Check sheet for the modelled part. Datum: model origin and axes. Units: mm. A direction names the side the tool comes from. Give positions to 0.01 mm unless a question says otherwise; leave off trailing zeros. Write each loop counter-clockwise with the first axis right and the second up, starting at its lowest first coordinate (ties: lowest second). Pieces come first, ordered by that corner, then holes. Notation, with made-up numbers: M 67.25,-3.75 L 81.25,-3.75 A20 ccw 81.25,25.25 Z; hole C 24,-20 d1. An arc over 180 degrees is marked long. Use CSV: the item, a comma, the result in double quotes. Start each with the question number.
1. Scan lines: line 1 (Z direction, x = -15, y = -0.05); line 2 (X direction, y = -0.25, z = -29); line 3 (X direction, y = -0.3, z = -2). Record each from-to range of solid material in increasing order.
2. Cross-section at C-C, the plane y = 0.45. Enter the section's corners in (x, z).
3. Cross-section at B-B, the plane z = -35. Enter the section's corners in (x, y), and give its area (3 significant figures).
4. Cross-section at D-D, the plane z = 21. Enter the section's corners in (x, y).
5. Access from +Z, -Z, +X, -X, +Y, -Y to the whole of each face (thin tool, end or side, straight path). Record for faces 1 (the face through (-0.476, 0.493, 49.697)), 2 (the face through (27.75, -0.25, 34.94)), 3 (the face through (-5.43, -0.25, 46.97)).
6. Mould release check, pull along Z, two halves, no side actions. Record for faces 4 (the face through (-2, -0.5, 1)), 5 (the face through (23.274, -0.092, -0.447)), 6 (the face through (0.5, 0.5, -49.8)): +Z half, -Z half, draft (parallel to the pull), parting line (faces both ways), or undercut.
7. Cross-section at A-A, the plane x = -23. Enter the section's corners in (y, z).
8. Depth check by flat-ended pin: P1, Ø5, axis at x = 30.5, z = -35, coming from the -Y side; P2, Ø0.6, axis at y = -0.5, z = 31.5, coming from the +X side; P3, Ø8, axis at x = 26.5, z = -6, coming from the -Y side. Enter the tip coordinate at first touch or a pass-through.
from build123d import *

# Parameters (mm, degrees)
EXTRUDE_1_DEPTH     = 1
CUT_EXTRUDE_1_REACH = 65.213
SKETCH_3_R          = 1.5
EXTRUDE_2_DEPTH     = 0.5
FILLET_1_R          = 2


with BuildPart() as part:
    # 스케치2 → 보스-돌출1 (new body)
    with BuildSketch(Plane(origin=(0, 0, 0), x_dir=(1, 0, 0), z_dir=(0, 1, 0))):
        Polygon((34, 30), (34, 53.281300489), (-34, 46.211993558), (-34, -46.211993558), (34, -53.281300489), (34, -30), (24, -30), (24, 30), align=None)
    extrude(amount=EXTRUDE_1_DEPTH)

    # 스케치3 → 컷-돌출1 (cut, up to next)
    with BuildSketch(Plane.XZ, mode=Mode.PRIVATE) as cut_extrude_1_sk1:
        with Locations(Location((-23, 43.836695157, 0), (0, 0, 270))):
            Circle(SKETCH_3_R)
    cut_extrude_1_tool1 = extrude(cut_extrude_1_sk1.sketch, amount=-CUT_EXTRUDE_1_REACH, mode=Mode.PRIVATE) & part.part
    # 스케치3 → 컷-돌출1 (cut, up to next)
    with BuildSketch(Plane.XZ, mode=Mode.PRIVATE) as cut_extrude_1_sk2:
        with Locations(Location((12, 47.475309018, 0), (0, 0, 270))):
            Circle(SKETCH_3_R)
    cut_extrude_1_tool2 = extrude(cut_extrude_1_sk2.sketch, amount=-CUT_EXTRUDE_1_REACH, mode=Mode.PRIVATE) & part.part
    # 스케치3 → 컷-돌출1 (cut, up to next)
    with BuildSketch(Plane.XZ, mode=Mode.PRIVATE) as cut_extrude_1_sk3:
        with Locations(Location((30.5, 35, 0), (0, 0, 270))):
            Circle(SKETCH_3_R)
    cut_extrude_1_tool3 = extrude(cut_extrude_1_sk3.sketch, amount=-CUT_EXTRUDE_1_REACH, mode=Mode.PRIVATE) & part.part
    # 스케치3 → 컷-돌출1 (cut, up to next)
    with BuildSketch(Plane.XZ, mode=Mode.PRIVATE) as cut_extrude_1_sk4:
        with Locations(Location((30.5, -35, 0), (0, 0, 270))):
            Circle(SKETCH_3_R)
    cut_extrude_1_tool4 = extrude(cut_extrude_1_sk4.sketch, amount=-CUT_EXTRUDE_1_REACH, mode=Mode.PRIVATE) & part.part
    # 스케치3 → 컷-돌출1 (cut, up to next)
    with BuildSketch(Plane.XZ, mode=Mode.PRIVATE) as cut_extrude_1_sk5:
        with Locations(Location((-23, -43.836695157, 0), (0, 0, 270))):
            Circle(SKETCH_3_R)
    cut_extrude_1_tool5 = extrude(cut_extrude_1_sk5.sketch, amount=-CUT_EXTRUDE_1_REACH, mode=Mode.PRIVATE) & part.part
    # 스케치3 → 컷-돌출1 (cut, up to next)
    with BuildSketch(Plane.XZ, mode=Mode.PRIVATE) as cut_extrude_1_sk6:
        with Locations(Location((12, -47.475309018, 0), (0, 0, 270))):
            Circle(SKETCH_3_R)
    cut_extrude_1_tool6 = extrude(cut_extrude_1_sk6.sketch, amount=-CUT_EXTRUDE_1_REACH, mode=Mode.PRIVATE) & part.part
    add(cut_extrude_1_tool1.solids().sort_by_distance((-23, 0, 43.836695))[0], mode=Mode.SUBTRACT)
    add(cut_extrude_1_tool2.solids().sort_by_distance((12, 0, 47.475309))[0], mode=Mode.SUBTRACT)
    add(cut_extrude_1_tool3.solids().sort_by_distance((30.5, 0, 35))[0], mode=Mode.SUBTRACT)
    add(cut_extrude_1_tool4.solids().sort_by_distance((30.5, 0, -35))[0], mode=Mode.SUBTRACT)
    add(cut_extrude_1_tool5.solids().sort_by_distance((-23, 0, -43.836695))[0], mode=Mode.SUBTRACT)
    add(cut_extrude_1_tool6.solids().sort_by_distance((12, 0, -47.475309))[0], mode=Mode.SUBTRACT)

    # 스케치4 → 보스-돌출2 (add)
    with BuildSketch(Plane.XZ):
        with BuildLine():
            Line((-34, 44.000136968), (-34, -44.000136968))
            Line((-34, -44.000136968), (-25.869682763, -44.845367968))
            Line((-25.869682763, -44.845367968), (-25.735258708, -43.552336579))
            ThreePointArc((-25.735258708, -43.552336579), (-22.715641421, -41.101436449), (-20.264741292, -44.121053736))
            Line((-20.264741292, -44.121053736), (-20.399165347, -45.414085125))
            Line((-20.399165347, -45.414085125), (9.130317237, -48.483981829))
            Line((9.130317237, -48.483981829), (9.264741292, -47.19095044))
            ThreePointArc((9.264741292, -47.19095044), (12.284358579, -44.740050311), (14.735258708, -47.759667597))
            Line((14.735258708, -47.759667597), (14.600834653, -49.052698986))
            Line((14.600834653, -49.052698986), (31.8, -50.840731027))
            Line((31.8, -50.840731027), (31.8, -37.75))
            Line((31.8, -37.75), (30.5, -37.75))
            ThreePointArc((30.5, -37.75), (27.75, -35), (30.5, -32.25))
            Line((30.5, -32.25), (31.8, -32.25))
            Line((31.8, -32.25), (31.8, -30))
            Line((31.8, -30), (24, -30))
            Line((24, -30), (24, 30))
            Line((24, 30), (31.8, 30))
            Line((31.8, 30), (31.8, 32.25))
            Line((31.8, 32.25), (30.5, 32.25))
            ThreePointArc((30.5, 32.25), (27.75, 35), (30.5, 37.75))
            Line((30.5, 37.75), (31.8, 37.75))
            Line((31.8, 37.75), (31.8, 50.840731027))
            Line((31.8, 50.840731027), (14.600834653, 49.052698986))
            Line((14.600834653, 49.052698986), (14.735258708, 47.759667597))
            ThreePointArc((14.735258708, 47.759667597), (12.284358579, 44.740050311), (9.264741292, 47.19095044))
            Line((9.264741292, 47.19095044), (9.130317237, 48.483981829))
            Line((9.130317237, 48.483981829), (-20.399165347, 45.414085125))
            Line((-20.399165347, 45.414085125), (-20.264741292, 44.121053736))
            ThreePointArc((-20.264741292, 44.121053736), (-22.715641421, 41.101436449), (-25.735258708, 43.552336579))
            Line((-25.735258708, 43.552336579), (-25.869682763, 44.845367968))
            Line((-25.869682763, 44.845367968), (-34, 44.000136968))
        make_face()
    extrude(amount=EXTRUDE_2_DEPTH)

    # 필렛1
    # the kernel refuses this fillet: 2 mm, written as the material it takes off along each edge
    with BuildSketch(Plane(origin=(36.641229183, -0.5, -30), x_dir=(0, 0, -1), z_dir=(-1, 0, 0)), Plane(origin=(24, -0.5, 30), x_dir=(0, 0, 1), z_dir=(1, 0, 0))) as fillet_1_piece_1:
        with BuildLine():
            CenterArc((1.936491673, -2), FILLET_1_R, 90, 75.522487814)
            Line((0, -1.5), (-0.038729833, -1.49))
            ThreePointArc((-0.038729833, -1.49), (-0.04, -0.75), (-0.04, 0))
            Line((-0.04, 0), (0, 0.04))
            Line((0, 0.04), (1.936491673, 0.04))
            Line((1.936491673, 0.04), (1.936491673, 0))
        make_face()
    extrude(amount=12.641229183, mode=Mode.SUBTRACT)
    with BuildSketch(Plane(origin=(24, -0.5, -30), x_dir=(-1, 0, 0), z_dir=(0, 0, 1))) as fillet_1_piece_2:
        with BuildLine():
            CenterArc((1.936491673, -2), FILLET_1_R, 90, 75.522487814)
            Line((0, -1.5), (-0.038729833, -1.49))
            ThreePointArc((-0.038729833, -1.49), (-0.04, -0.75), (-0.04, 0))
            Line((-0.04, 0), (0, 0.04))
            Line((0, 0.04), (1.936491673, 0.04))
            Line((1.936491673, 0.04), (1.936491673, 0))
        make_face()
    extrude(amount=60, mode=Mode.SUBTRACT)
    with BuildSketch(Plane(origin=(36.641229183, -0.5, -30), x_dir=(0, 0, -1), z_dir=(-1, 0, 0))) as fillet_1_piece_3a_section:
        with BuildLine():
            CenterArc((1.936491673, -2), FILLET_1_R, 90, 75.522487814)
            Line((0, -1.5), (-0.038729833, -1.49))
            ThreePointArc((-0.038729833, -1.49), (-0.04, -0.75), (-0.04, 0))
            Line((-0.04, 0), (0, 0.04))
            Line((0, 0.04), (1.936491673, 0.04))
            Line((1.936491673, 0.04), (1.936491673, 0))
        make_face()
    fillet_1_piece_3a = extrude(amount=17.482458366, mode=Mode.PRIVATE)
    fillet_1_piece_3a = split(fillet_1_piece_3a, bisect_by=Plane(origin=(24, -0.120816489, -30.456288202), z_dir=(-1, 0, 0)), keep=Keep.TOP, mode=Mode.PRIVATE)
    with BuildSketch(Plane(origin=(24, -0.5, -34.841229183), x_dir=(-1, 0, 0), z_dir=(0, 0, 1))) as fillet_1_piece_3b_section:
        with BuildLine():
            CenterArc((1.936491673, -2), FILLET_1_R, 90, 75.522487814)
            Line((0, -1.5), (-0.038729833, -1.49))
            ThreePointArc((-0.038729833, -1.49), (-0.04, -0.75), (-0.04, 0))
            Line((-0.04, 0), (0, 0.04))
            Line((0, 0.04), (1.936491673, 0.04))
            Line((1.936491673, 0.04), (1.936491673, 0))
        make_face()
    fillet_1_piece_3b = extrude(amount=64.841229183, mode=Mode.PRIVATE)
    fillet_1_piece_3b = split(fillet_1_piece_3b, bisect_by=Plane(origin=(23.543711798, -0.120816489, -30), z_dir=(0, 0, -1)), keep=Keep.TOP, mode=Mode.PRIVATE)
    fillet_1_piece_3 = fillet_1_piece_3a & fillet_1_piece_3b
    add(fillet_1_piece_3, mode=Mode.SUBTRACT)
    with BuildSketch(Plane(origin=(24, -0.5, -30), x_dir=(-1, 0, 0), z_dir=(0, 0, 1))) as fillet_1_piece_4a_section:
        with BuildLine():
            CenterArc((1.936491673, -2), FILLET_1_R, 90, 75.522487814)
            Line((0, -1.5), (-0.038729833, -1.49))
            ThreePointArc((-0.038729833, -1.49), (-0.04, -0.75), (-0.04, 0))
            Line((-0.04, 0), (0, 0.04))
            Line((0, 0.04), (1.936491673, 0.04))
            Line((1.936491673, 0.04), (1.936491673, 0))
        make_face()
    fillet_1_piece_4a = extrude(amount=64.841229183, mode=Mode.PRIVATE)
    fillet_1_piece_4a = split(fillet_1_piece_4a, bisect_by=Plane(origin=(23.543711798, -0.120816489, 30), z_dir=(0, 0, 1)), keep=Keep.TOP, mode=Mode.PRIVATE)
    with BuildSketch(Plane(origin=(19.158770817, -0.5, 30), x_dir=(0, 0, 1), z_dir=(1, 0, 0))) as fillet_1_piece_4b_section:
        with BuildLine():
            CenterArc((1.936491673, -2), FILLET_1_R, 90, 75.522487814)
            Line((0, -1.5), (-0.038729833, -1.49))
            ThreePointArc((-0.038729833, -1.49), (-0.04, -0.75), (-0.04, 0))
            Line((-0.04, 0), (0, 0.04))
            Line((0, 0.04), (1.936491673, 0.04))
            Line((1.936491673, 0.04), (1.936491673, 0))
        make_face()
    fillet_1_piece_4b = extrude(amount=17.482458366, mode=Mode.PRIVATE)
    fillet_1_piece_4b = split(fillet_1_piece_4b, bisect_by=Plane(origin=(24, -0.120816489, 30.456288202), z_dir=(-1, 0, 0)), keep=Keep.TOP, mode=Mode.PRIVATE)
    fillet_1_piece_4 = fillet_1_piece_4a & fillet_1_piece_4b
    add(fillet_1_piece_4, mode=Mode.SUBTRACT)


solid = part.part
Worked answers:
1,line 1,"z = -45.98 to 45.98"
1,line 2,"x = -34 to 23.03"
1,line 3,"x = -34 to 22.94"
2,outline,"M -34,-46.21 L 34,-53.28 L 34,-30.23 L 23.77,-30.23 L 23.77,30.23 L 34,30.23 L 34,53.28 L -34,46.21 Z; hole C -23,-43.84 d3; hole C -23,43.84 d3; hole C 12,-47.48 d3; hole C 12,47.48 d3; hole C 30.5,-35 d3; hole C 30.5,35 d3"
3,outline,"M -34,-0.5 L 27.75,-0.5 L 27.75,0 L 29,0 L 29,1 L -34,1 Z; M 32,0 L 34,0 L 34,1 L 32,1 Z"
3,area,"95.9 mm^2"
4,outline,"M -34,-0.5 L 22.06,-0.5 A2 ccw 24,1 L -34,1 Z"
5,face 1,"+Z, -X, +Y, -Y"
5,face 2,"+X, -Y"
5,face 3,"+Z, -X, -Y"
6,face 4,"draft"
6,face 5,"undercut"
6,face 6,"-Z half"
7,outline,"M -0.5,-41.09 L 0,-41.09 L 0,-42.34 L 1,-42.34 L 1,42.34 L 0,42.34 L 0,41.09 L -0.5,41.09 Z; M 0,-47.36 L 1,-47.36 L 1,-45.34 L 0,-45.34 Z; M 0,45.34 L 1,45.34 L 1,47.36 L 0,47.36 Z"
8,P1,"stops at y = 0"
8,P2,"stops at x = 31.8"
8,P3,"stops at y = -0.45"
